Here's how the part is built. I have some questions about the finished solid (model axes, mm). Face numbers are marked on the shaded views. A direction names the side the tool comes from. Coordinates: 2 decimals unless noted, no trailing zeros. Order: outer loops, then holes, each group sorted by start corner. A loop starts at its lowest first (then second) coordinate and runs counter-clockwise, first axis right, second up. Notation, with made-up numbers: (-16.5, -9.75) -> (26.5, -9.75) arc R22 cw to (26.5, 28.25) -> close; hole circle Ø6 at (87, -9). An arc over 180 degrees is marked (long way). One line per item, written item: value. Start each with the question number.
```python
from build123d import *

# Parameters (mm, degrees)
EXTRUDE_1_DEPTH            = 15
SKETCH_2_W                 = 3
SKETCH_2_H                 = 19
SKETCH_2_W_2               = 10
SKETCH_2_H_2               = 3
CUT_EXTRUDE_1_DEPTH        = 16
SKETCH_3_W                 = 18.5
SKETCH_3_H                 = 3
SKETCH_3_W_2               = 8.5
CUT_EXTRUDE_3_DEPTH        = 8
HOLE_WIZARD_M31_AT_2_COUNT = 2
HOLE_WIZARD_M31_AT_2_PITCH = 22
HOLE_WIZARD_M31_AT_3_COUNT = 2
HOLE_WIZARD_M31_AT_3_PITCH = 11
CUT_EXTRUDE_4_REACH        = 23.5


with BuildPart() as part:
    # Эскиз1 → Бобышка-Вытянуть1 (new body)
    with BuildSketch(Plane.XY):
        Polygon((-1.5, 0), (-1.5, 22), (-20, 22), (-20, 25), (20, 25), (20, 22), (1.5, 22), (1.5, 0), align=None)
    extrude(amount=EXTRUDE_1_DEPTH)

    # Эскиз2 → Вырез-Вытянуть1 (cut, through all)
    with BuildSketch(Plane.XY.offset(15)):
        with Locations((0, 9.5)):
            Rectangle(SKETCH_2_W, SKETCH_2_H)
        with Locations((15, 23.5)):
            Rectangle(SKETCH_2_W_2, SKETCH_2_H_2)
    extrude(amount=-CUT_EXTRUDE_1_DEPTH, mode=Mode.SUBTRACT)

    # Эскиз3 → Вырез-Вытянуть3 (cut)
    with BuildSketch(Plane.XY.offset(15)):
        with Locations((-10.75, 23.5)):
            Rectangle(SKETCH_3_W, SKETCH_3_H)
        with Locations((5.75, 23.5)):
            Rectangle(SKETCH_3_W_2, SKETCH_3_H)
    extrude(amount=-CUT_EXTRUDE_3_DEPTH, mode=Mode.SUBTRACT)

    # Эскиз4 → Отверстие с зазором M31 (revolve, cut)
    with BuildSketch(Plane(origin=(-15.5, 22, 4), x_dir=(0, 0, -1), z_dir=(1, 0, 0))):
        Polygon((0, 0), (0, 3), (1.725, 3), (1.6, 2.875), (1.6, 0.125), (1.725, 0), align=None)
    hole_wizard_m31 = revolve(axis=Axis((-15.5, 15.65, 4), (0, 1, 0)), mode=Mode.SUBTRACT)

    # Отверстие с зазором M31 at 2: Отверстие с зазором M31 ×2
    with Locations(*[(i * HOLE_WIZARD_M31_AT_2_PITCH, 0, 0) for i in range(1, HOLE_WIZARD_M31_AT_2_COUNT)]):
        add(hole_wizard_m31, mode=Mode.SUBTRACT)

    # Отверстие с зазором M31 at 3: Отверстие с зазором M31 ×2
    with Locations(*[(i * HOLE_WIZARD_M31_AT_3_PITCH, 0, 0) for i in range(1, HOLE_WIZARD_M31_AT_3_COUNT)]):
        add(hole_wizard_m31, mode=Mode.SUBTRACT)

    # Эскиз6 → Вырез-Вытянуть4 (cut, up to next)
    with BuildSketch(Plane(origin=(1.5, 0, 0), x_dir=(0, 0, -1), z_dir=(1, 0, 0)), mode=Mode.PRIVATE) as cut_extrude_4_sk1:
        with BuildLine():
            Line((-11.85, 23.65), (-10.15, 23.65))
            ThreePointArc((-10.15, 23.65), (-8.5, 22), (-10.15, 20.35))
            Line((-10.15, 20.35), (-11.85, 20.35))
            ThreePointArc((-11.85, 20.35), (-13.5, 22), (-11.85, 23.65))
        make_face()
    cut_extrude_4_tool1 = extrude(cut_extrude_4_sk1.sketch, amount=-CUT_EXTRUDE_4_REACH, mode=Mode.PRIVATE) & part.part
    add(cut_extrude_4_tool1.solids().sort_by_distance((1.5, 22, 11))[0], mode=Mode.SUBTRACT)


solid = part.part
```
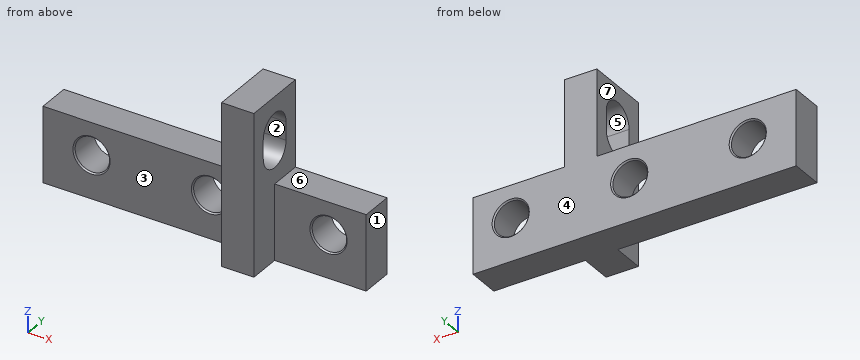
Q1. Imagine slicing it at D-D (z = 10.5). Write out the boundary of the cut face in (x, y), plus the area to 3 significant figures.
Q2. Imagine slicing it at A-A (y = 23). Write out the boundary of the cut face in (x, z), plus the area to 3 significant figures.
Q3. For the marked faces 5, 6 and 7, which set-ups out of +Z, -Z, +X, -X, +Y, -Y let a thin tool reach every point of the face, with its end or its side?
Q4. I need wall thicknesses on line 1 (X direction, y = 24.1, z = 4); line 2 (Z direction, x = 6.5, y = 22.9); line 3 (Z direction, x = -8.5, y = 23.8). Which ranges of each line are inside material? Lowest first, please.
Q5. Imagine slicing it at B-B (z = 4). Count the separate pieces of the cut face and the enclosed holes in it, plus the area to 3 significant figures.
Q6. For P1, Ø3.5, axis at x = -11.5, y = 24, coming from the +Z side; P2, Ø5.5, axis at x = 5, z = 2.5, coming from the -Y side; P3, Ø6, axis at x = -15.5, z = 12.5, coming from the -Y side (3 decimals); P4, Ø3, axis at y = 21.5, z = 10.5, coming from the +X side, each with a flat end and sliding along its axis, tell me the tip position at first contact or that it passes through.
Q7. If we mould it in two halves opening along Y, with no side actions, what happens to the marked faces 1, 2, 3 and 4? For each: +Y half, -Y half, draft (parallel to the pull), parting line (faces both ways), or undercut.
Q8. Imagine slicing it at C-C (x = -4.5). Write out the boundary of the cut face in (y, z) (3 decimals).
Completed:
1. outline: (-1.5, 19) -> (1.5, 19) -> (1.5, 20.35) -> (-1.5, 20.35) -> close; (-1.5, 23.65) -> (1.5, 23.65) -> (1.5, 25) -> (-1.5, 25) -> close
1. area: 8.10 mm2
2. outline: (-20, 0) -> (10, 0) -> (10, 7) -> (1.5, 7) -> (1.5, 8.84) -> (-1.5, 8.84) -> (-1.5, 7) -> (-20, 7) -> close; (-1.5, 13.16) -> (1.5, 13.16) -> (1.5, 15) -> (-1.5, 15) -> close; hole circle Ø3.2 at (-15.5, 4); hole circle Ø3.2 at (-4.5, 4); hole circle Ø3.2 at (6.5, 4)
2. area: 197 mm2
3. face 5: +X, -X
3. face 6: +Z, +X, +Y, -Y
3. face 7: +Z, -X, -Y
4. line 1: x = -20 to -17.1, -13.9 to -6.1, -2.9 to 4.9, 8.1 to 10
4. line 2: z = 0 to 2.4, 5.6 to 7
4. line 3: z = 0 to 7
5. separate pieces: 4
5. enclosed holes: 0
5. area: 70.1 mm2
6. P1: stops at z = 7
6. P2: stops at y = 22
6. P3: passes through
6. P4: stops at x = 1.5
7. face 1: draft
7. face 2: undercut
7. face 3: -Y half
7. face 4: +Y half
8. outline: (22, 0) -> (25, 0) -> (25, 2.275) -> (24.875, 2.4) -> (22.125, 2.4) -> (22, 2.275) -> close; (22, 5.725) -> (22.125, 5.6) -> (24.875, 5.6) -> (25, 5.725) -> (25, 7) -> (22, 7) -> close
